The listing builds one solid part. Answer for the finished solid, in the listing's coordinates (mm). A direction names the side the tool comes from. Round coordinates to 2 decimals unless told otherwise and drop trailing zeros. Write each loop counter-clockwise with the first axis right and the second up, starting at its lowest first coordinate (ties: lowest second). Pieces come first, ordered by that corner, then holes.
from build123d import *

# Parameters (mm, degrees)
SKETCH1_R           = 3.5
BOSS_EXTRUDE1_DEPTH = 1.5


with BuildPart() as part:
    # Sketch1 → Boss-Extrude1 (new, symmetric)
    with BuildSketch(Plane(origin=(0, 0, 0), x_dir=(1, 0, 0), z_dir=(0, 1, 0))):
        with BuildLine():
            Line((-1.7, 28.25), (1.7, 28.25))
            Line((1.7, 28.25), (1.7, 32.75))
            Line((1.7, 32.75), (5.003947629, 32.75))
            ThreePointArc((5.003947629, 32.75), (13.711796564, 13.711796564), (32.75, 5.003947629))
            Line((32.75, 5.003947629), (32.75, 1.7))
            Line((32.75, 1.7), (28.25, 1.7))
            Line((28.25, 1.7), (28.25, -1.7))
            Line((28.25, -1.7), (32.75, -1.7))
            Line((32.75, -1.7), (32.75, -5.003947629))
            ThreePointArc((32.75, -5.003947629), (13.711796564, -13.711796564), (5.003947629, -32.75))
            Line((5.003947629, -32.75), (1.7, -32.75))
            Line((1.7, -32.75), (1.7, -28.25))
            Line((1.7, -28.25), (-1.7, -28.25))
            Line((-1.7, -28.25), (-1.7, -32.75))
            Line((-1.7, -32.75), (-5.003947629, -32.75))
            ThreePointArc((-5.003947629, -32.75), (-13.711796564, -13.711796564), (-32.75, -5.003947629))
            Line((-32.75, -5.003947629), (-32.75, -1.7))
            Line((-32.75, -1.7), (-28.25, -1.7))
            Line((-28.25, -1.7), (-28.25, 1.7))
            Line((-28.25, 1.7), (-32.75, 1.7))
            Line((-32.75, 1.7), (-32.75, 5.003947629))
            ThreePointArc((-32.75, 5.003947629), (-13.711796564, 13.711796564), (-5.003947629, 32.75))
            Line((-5.003947629, 32.75), (-1.7, 32.75))
            Line((-1.7, 32.75), (-1.7, 28.25))
        make_face()
        with Locations(Location((0, 0, 0), (0, 0, 270))):
            Circle(SKETCH1_R, mode=Mode.SUBTRACT)
    extrude(amount=BOSS_EXTRUDE1_DEPTH, both=True)


solid = part.part
1. Section B-B on z = 0 is taken. Determine the outline of the cut face in (x, y), plus the area to 4 significant figures.
Geometry says:
outline: (-28.25, -1.5) - (-3.5, -1.5) - (-3.5, 1.5) - (-28.25, 1.5) - close; (3.5, -1.5) - (28.25, -1.5) - (28.25, 1.5) - (3.5, 1.5) - close
area: 148.5 mm2
2. Section D-D on z = -15 is taken. Determine the outline of the cut face in (x, y).
Geometry says:
outline: (-12.5, -1.5) - (12.5, -1.5) - (12.5, 1.5) - (-12.5, 1.5) - close
3. A tool of negligible diameter and unlimited length cuts with its end or side. For faces 1 (the face through (1.7, 0, -30)), 2 (the face through (1.7, 0, 31)), 3 (the face through (-31, 0, 1.7)), 4 (the face through (30, 0, 1.7)), from which of +Z, -Z, +X, -X, +Y, -Y can it reach the whole face along a straight path? Write none if from no direction.
Geometry says:
face 1: -Z, +Y, -Y
face 2: +Z, +Y, -Y
face 3: -X, +Y, -Y
face 4: +X, +Y, -Y
4. Straight lines are drawn through the part: line 1 along X through (y, z) = (-0.65, 0); line 2 along X through (y, z) = (-0.9, 20.5); line 3 along X through (y, z) = (0.15, -30). For each, find the intervals that lie inside material, in ascending order.
Geometry says:
line 1: x = -28.25 to -3.5, 3.5 to 28.25
line 2: x = -8.62 to 8.62
line 3: x = -5.33 to -1.7, 1.7 to 5.33
5. Given pin 1 (1.5 mm diameter, centred on y = -0.5, z = -29.5, fed in from -X); pin 2 (0.9 mm diameter, centred on x = -30.5, y = -0.5, fed in from -Z); pin 3 (1 mm diameter, centred on y = 0, z = 9.5, fed in from -X); pin 4 (12 mm diameter, centred on x = 26, z = -12.5, fed in from -Y), each flat-ended and moving along its own axis, determine where each tip first touches the part or whether it passes through.
Geometry says:
pin 1: stops at x = -5.57
pin 2: stops at z = -5.32
pin 3: stops at x = -19.83
pin 4: stops at y = -1.5
6. Section C-C on y = -0.4 is taken. Determine the outline of the cut face in (x, z) (3 decimals), plus the area to 3 significant figures.
Geometry says:
outline: (-32.75, -5.004) arc R30 cw to (-5.004, -32.75) - (-1.7, -32.75) - (-1.7, -28.25) - (1.7, -28.25) - (1.7, -32.75) - (5.004, -32.75) arc R30 cw to (32.75, -5.004) - (32.75, -1.7) - (28.25, -1.7) - (28.25, 1.7) - (32.75, 1.7) - (32.75, 5.004) arc R30 cw to (5.004, 32.75) - (1.7, 32.75) - (1.7, 28.25) - (-1.7, 28.25) - (-1.7, 32.75) - (-5.004, 32.75) arc R30 cw to (-32.75, 5.004) - (-32.75, 1.7) - (-28.25, 1.7) - (-28.25, -1.7) - (-32.75, -1.7) - close; hole circle Ø7 at (0, 0)
area: 1,870 mm2
7. Section A-A on x = 0 is taken. Determine the outline of the cut face in (y, z), plus the area to 4 significant figures.
Geometry says:
outline: (-1.5, -28.25) - (1.5, -28.25) - (1.5, -3.5) - (-1.5, -3.5) - close; (-1.5, 3.5) - (1.5, 3.5) - (1.5, 28.25) - (-1.5, 28.25) - close
area: 148.5 mm2
8. For a pull along Z with two mould halves and no side action, classify faces 5 (the face through (-3, 0, -32.75)), 6 (the face through (28.25, 0, 0)), 7 (the face through (-7, -1.5, 0)) as released by +Z, released by -Z, zero draft, split by the parting line, or undercut.
Geometry says:
face 5: released by -Z
face 6: undercut
face 7: zero draft
